Read the model definition and answer for the solid it produces. Units are mm, in the model's axes. A direction names the side the tool comes from. Give positions to 0.01 mm unless a question says otherwise; leave off trailing zeros. Write each loop counter-clockwise with the first axis right and the second up, starting at its lowest first coordinate (ties: lowest second). Pieces come first, ordered by that corner, then holes.
```python
from build123d import *

# Parameters (mm, degrees)
F0_R      = 38.1
F1_DEPTH  = 25.4
F2_R      = 31.75
F3_DEPTH  = 25.4
F4_R      = 25.4
F5_DEPTH  = 50.8
F6_R      = 6.35
F7_DEPTH  = 53.594
F7_FACE_R = 6.35
F10_R     = 5.3624799473
F11_DEPTH = 53.848
F9_R      = 5.3624799473
F12_DEPTH = 53.848


# Not quite as in the source:
# - an extrude whose draft closes it to a point is written as a loft to that point


with BuildPart() as f1:
    # F0 (on Top) → F1 (new body)
    with BuildSketch(Plane.XY):
        Circle(F0_R)
    extrude(amount=F1_DEPTH)

    # F2 (on Top) → F3 (join)
    with BuildSketch(Plane.XY):
        Circle(F2_R)
    extrude(amount=-F3_DEPTH)

    # F4 (on Top) → F5 (join)
    with BuildSketch(Plane.XY):
        Circle(F4_R)
    extrude(amount=-F5_DEPTH)

    # F6 (on Top) → F7 (join)
    with BuildSketch(Plane.XY):
        Circle(F6_R)
    extrude(amount=-F7_DEPTH)

    # F7_face (on face) → F8 section 0
    with BuildSketch(Plane(origin=(0, 0, -53.594), x_dir=(1, 0, 0), z_dir=(0, 0, -1)), mode=Mode.PRIVATE) as f8_s0:
        Circle(F7_FACE_R)
    loft([f8_s0.sketch, Vertex(0, 0, -98.7765977371)], ruled=True)

    # F10 (on Top) → F11 (join)
    with BuildSketch(Plane.XY):
        with Locations((0, 17.3083227128)):
            Circle(F10_R)
    extrude(amount=-F11_DEPTH)

    # F9 (on Top) → F12 (join)
    with BuildSketch(Plane.XY):
        with Locations((0, -17.9224163294)):
            Circle(F9_R)
    extrude(amount=-F12_DEPTH)


solid = f1.part
```
Item 1: Which of the six approach directions +Z, -Z, +X, -X, +Y, -Y give full straight-line access (tool end or side, diameter ignored) to faces 1 (the flat face through (-14.3, 21.3, -25.4)), 2 (the flat face through (-1, 1, 25.4)), 3 (the flat face through (0, -18, -53.848)), 4 (the flat face through (0, 17, -53.848)), 5 (the cylindrical face through (-30.235, -23.183, 12.522))?
Result set:
face 1: -Z
face 2: +Z, +X, -X, +Y, -Y
face 3: -Z, +X, -X, -Y
face 4: -Z, +X, -X, +Y
face 5: +Z, -Z
Item 2: Section A-A (x = 15) is taken. Write down the section's boundary in (y, z), and give its area (3 significant figures).
Result set:
outline: (-35.02, 0) - (-27.98, 0) - (-27.98, -25.4) - (-20.5, -25.4) - (-20.5, -50.8) - (20.5, -50.8) - (20.5, -25.4) - (27.98, -25.4) - (27.98, 0) - (35.02, 0) - (35.02, 25.4) - (-35.02, 25.4) - close
area: 4,240 mm2
Item 3: Section C-C (z = -15) is taken. Write down the section's boundary in (x, y).
Result set:
outline: circle Ø63.5 at (0, 0)
Item 4: Section B-B (y = 27) is taken. Write down the section's boundary in (x, z), and give its area (3 significant figures).
Result set:
outline: (-26.88, 0) - (-16.71, 0) - (-16.71, -25.4) - (16.71, -25.4) - (16.71, 0) - (26.88, 0) - (26.88, 25.4) - (-26.88, 25.4) - close
area: 2,210 mm2
Item 5: Find the intervals of material crossed by line 1 along Y through (x, z) = (0.5, -52.5); line 2 along Z through (x, y) = (20, -2); line 3 along Z through (x, y) = (-11, 23.5), in increasing order.
Result set:
line 1: y = -23.26 to -12.58, -6.33 to 6.33, 11.97 to 22.65
line 2: z = -50.8 to 25.4
line 3: z = -25.4 to 25.4
Item 6: Section D-D (x = -19) is taken. Write down the section's boundary in (y, z).
Result set:
outline: (-33.02, 0) - (-25.44, 0) - (-25.44, -25.4) - (-16.86, -25.4) - (-16.86, -50.8) - (16.86, -50.8) - (16.86, -25.4) - (25.44, -25.4) - (25.44, 0) - (33.02, 0) - (33.02, 25.4) - (-33.02, 25.4) - close
Item 7: Each of these flat-tipped pins is pushed along its axis until it touches: pin 1 Ø1.5 at (y, z) = (-18.5, 13) entering from -X; pin 2 Ø5 at (x, y) = (-16.5, -16) entering from -Z; pin 3 Ø3 at (x, y) = (2, -19) entering from -Z. Where does it stop, or does it pass through?
Result set:
pin 1: stops at x = -33.71
pin 2: stops at z = -50.8
pin 3: stops at z = -53.85
